from build123d import *

# Parameters (mm, degrees)
CYLINDER066_R     = 2
CYLINDER066_DEPTH = 10
CYLINDER068_R     = 2
CYLINDER068_DEPTH = 10
CYLINDER067_R     = 2
CYLINDER067_DEPTH = 10
CYLINDER065_R     = 2
CYLINDER065_DEPTH = 10
BOX059_W          = 10
BOX059_H          = 24
BOX059_DEPTH      = 9.6
BOX055_W          = 10.4
BOX055_H          = 107.2
BOX055_DEPTH      = 5
BOX056_W          = 10.4
BOX056_H          = 107.2
BOX056_DEPTH      = 5
BOX054_W          = 10
BOX054_H          = 2
BOX054_DEPTH      = 130
BOX053_W          = 10
BOX053_H          = 2
BOX053_DEPTH      = 130
BOX052_W          = 2
BOX052_H          = 110
BOX052_DEPTH      = 130


with BuildPart() as rueck_loch002:
    # Cylinder066 → Cylinder066 (new body)
    with BuildSketch(Plane(origin=(-6, 5, 123), x_dir=(1, 0, 0), z_dir=(0, -1, 0))):
        Circle(CYLINDER066_R)
    extrude(amount=CYLINDER066_DEPTH)


with BuildPart() as rueck_loch004:
    # Cylinder068 → Cylinder068 (new body)
    with BuildSketch(Plane(origin=(-6, 115, 123), x_dir=(1, 0, 0), z_dir=(0, -1, 0))):
        Circle(CYLINDER068_R)
    extrude(amount=CYLINDER068_DEPTH)


with BuildPart() as rueck_loch003:
    # Cylinder067 → Cylinder067 (new body)
    with BuildSketch(Plane(origin=(-6, 115, 7), x_dir=(1, 0, 0), z_dir=(0, -1, 0))):
        Circle(CYLINDER067_R)
    extrude(amount=CYLINDER067_DEPTH)


with BuildPart() as obj1:
    # Cylinder065 → Cylinder065 (new body)
    with BuildSketch(Plane(origin=(-6, 5, 7), x_dir=(1, 0, 0), z_dir=(0, -1, 0))):
        Circle(CYLINDER065_R)
    extrude(amount=CYLINDER065_DEPTH)

    # Fusion033: union Rueck_Loch002, Rueck_Loch004, Rueck_Loch003
    add(rueck_loch002.part)
    add(rueck_loch004.part)
    add(rueck_loch003.part)


with BuildPart() as obj2:
    # Box059 → Box059 (new body)
    with BuildSketch(Plane(origin=(-5, 43, 34.2), x_dir=(1, 0, 0), z_dir=(0, 0, 1))):
        with Locations((5, 12)):
            Rectangle(BOX059_W, BOX059_H)
    extrude(amount=BOX059_DEPTH)


with BuildPart() as cube047:
    # Box055 → Box055 (new body)
    with BuildSketch(Plane(origin=(-10, 1.4, 0), x_dir=(1, 0, 0), z_dir=(0, 0, 1))):
        with Locations((5.2, 53.6)):
            Rectangle(BOX055_W, BOX055_H)
    extrude(amount=BOX055_DEPTH)


with BuildPart() as fusion024:
    # Box056 → Box056 (new body)
    with BuildSketch(Plane(origin=(-10, 1.4, 125), x_dir=(1, 0, 0), z_dir=(0, 0, 1))):
        with Locations((5.2, 53.6)):
            Rectangle(BOX056_W, BOX056_H)
    extrude(amount=BOX056_DEPTH)

    # Fusion024: union Cube047
    add(cube047.part)


with BuildPart() as cube046:
    # Box054 → Box054 (new body)
    with BuildSketch(Plane(origin=(-10, 108, 0), x_dir=(1, 0, 0), z_dir=(0, 0, 1))):
        with Locations((5, 1)):
            Rectangle(BOX054_W, BOX054_H)
    extrude(amount=BOX054_DEPTH)


with BuildPart() as cube045:
    # Box053 → Box053 (new body)
    with BuildSketch(Plane(origin=(-10, 0, 0), x_dir=(1, 0, 0), z_dir=(0, 0, 1))):
        with Locations((5, 1)):
            Rectangle(BOX053_W, BOX053_H)
    extrude(amount=BOX053_DEPTH)


with BuildPart() as obj3:
    # Box052 → Box052 (new body)
    with BuildSketch(Plane.XY):
        with Locations((1, 55)):
            Rectangle(BOX052_W, BOX052_H)
    extrude(amount=BOX052_DEPTH)

    # Fusion023: union Cube046, Cube045
    add(cube046.part)
    add(cube045.part)

    # Cut052: cut Fusion024
    add(fusion024.part, mode=Mode.SUBTRACT)

    # Cut054: cut obj2
    add(obj2.part, mode=Mode.SUBTRACT)

    # Cut062: cut obj1
    add(obj1.part, mode=Mode.SUBTRACT)


solid = obj3.part
Input: part model. Units: mm. Frame: model coordinates. A direction names the side the tool comes from. Give positions to 0.01 mm unless a question says otherwise; leave off trailing zeros. Write each loop counter-clockwise with the first axis right and the second up, starting at its lowest first coordinate (ties: lowest second). Pieces come first, ordered by that corner, then holes. Notation, with made-up numbers: (27, 75) -> (79, 75) arc R29 cw to (79, 111) -> close; hole circle Ø6 at (74.25, 37.25). An arc over 180 degrees is marked (long way). Use one line per item in the form item = value. Start each with the question number.
1) Set-up query: faces 4 (the flat face through (-5, 108.6, 127)), 5 (the flat face through (0, 54, 64)), 6 (the flat face through (-5, 108.6, 2)). Return all of +Z, -Z, +X, -X, +Y, -Y with unobstructed straight access to the full face (end or side cutting, diameter ignored); none if empty.
2) Ray query, probe 1 along Z at (x, y) = (-6, 109.35); probe 2 along Y at (x, z) = (-8.75, 34.5); probe 3 along X at (y, z) = (1.5, 123). Return the intervals inside material, ascending. Write a range as from..to.
3) Section query A-A on x = -1.5. Return the cut outline in (y, z).
4) Section query D-D on y = 9. Return the cut outline in (x, z).
5) Pin query (flat end, axial travel): pin 1 (8 mm diameter, centred on y = 13, z = 91.5, fed in from -X); pin 2 (5 mm diameter, centred on x = -4, y = 42, fed in from +Z); pin 3 (4 mm diameter, centred on y = 71.5, z = 2, fed in from -X); pin 4 (0.5 mm diameter, centred on x = -7, y = 2, fed in from +Z). Return the tip coordinate at first contact, or that it passes through.
6) Section query B-B on z = 123. Return the cut outline in (x, y), then the cut area to 3 significant figures.
7) Draft query along Y for faces 1 (the flat face through (-5, 1.4, 127)), 2 (the flat face through (-4, 0, 64)), 3 (the flat face through (2, 54, 64)). Return one class per face: pulls with the +Y half, pulls with the -Y half, needs draft (parallel to the pull), parting line crosses it, or undercut.
8) Section query C-C on z = 84.5. Return the cut outline in (x, y).
Outcome:
q1.face_4 = +Z, -X
q1.face_5 = +Z, -Z, -X
q1.face_6 = -Z, -X
q2.probe_1 = 0..5, 9..121, 125..130
q2.probe_2 = 0..2, 108..110
q2.probe_3 = -10..-8, -4..2
q3.outline = (0, 0) -> (1.4, 0) -> (1.4, 5) -> (2, 5) -> (2, 125) -> (1.4, 125) -> (1.4, 130) -> (0, 130) -> close; (108, 5) -> (108.6, 5) -> (108.6, 0) -> (110, 0) -> (110, 130) -> (108.6, 130) -> (108.6, 125) -> (108, 125) -> close
q4.outline = (0, 5) -> (0.4, 5) -> (0.4, 0) -> (2, 0) -> (2, 130) -> (0.4, 130) -> (0.4, 125) -> (0, 125) -> close
q5.pin_1 = 0
q5.pin_2 = through
q5.pin_3 = 0.4
q5.pin_4 = 125
q6.outline = (-10, 0) -> (-8, 0) -> (-8, 2) -> (-10, 2) -> close; (-10, 108) -> (-8, 108) -> (-8, 110) -> (-10, 110) -> close; (-4, 0) -> (2, 0) -> (2, 110) -> (-4, 110) -> (-4, 108) -> (0, 108) -> (0, 2) -> (-4, 2) -> close
q6.area = 244 mm^2
q7.face_1 = undercut
q7.face_2 = pulls with the -Y half
q7.face_3 = needs draft
q8.outline = (-10, 0) -> (2, 0) -> (2, 110) -> (-10, 110) -> (-10, 108) -> (0, 108) -> (0, 2) -> (-10, 2) -> close
